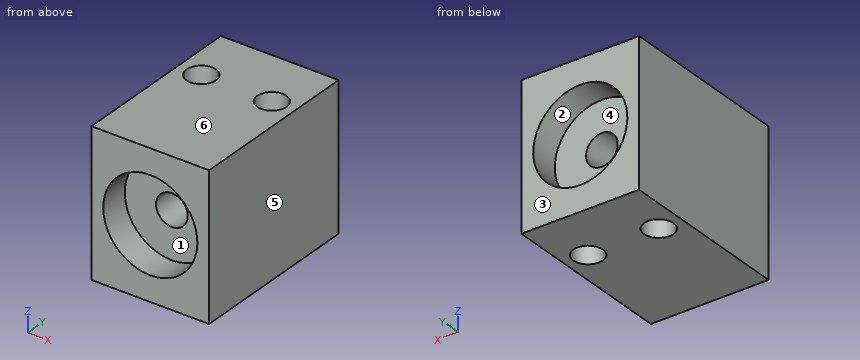
```python
from build123d import *

# Parameters (mm, degrees)
SKETCH1_W           = 20
SKETCH1_H           = 30
BOSS_EXTRUDE1_DEPTH = 12.25
SKETCH4_R           = 2.5
CUT_EXTRUDE1_DEPTH  = 25.5


with BuildPart() as part:
    # Sketch1 → Boss-Extrude1 (new body, symmetric)
    with BuildSketch(Plane.XY):
        Rectangle(SKETCH1_W, SKETCH1_H)
    extrude(amount=BOSS_EXTRUDE1_DEPTH, both=True)

    # Sketch3 → Cut-Revolve1 (revolve, cut)
    with BuildSketch(Plane(origin=(0, 0, 0), x_dir=(0, 0, -1), z_dir=(1, 0, 0))):
        Polygon((0, 15), (0, -15), (8, -15), (8, -10), (2.7, -10), (2.7, 10), (8, 10), (8, 15), align=None)
    revolve(axis=Axis((0, 15, 0), (0, -1, 0)), mode=Mode.SUBTRACT)

    # Sketch4 → Cut-Extrude1 (cut, through all)
    with BuildSketch(Plane(origin=(0, 0, -12.25), x_dir=(-1, 0, 0), z_dir=(0, 0, -1))):
        with Locations((-6, 5)):
            Circle(SKETCH4_R)
        with Locations((6, 5)):
            Circle(SKETCH4_R)
    extrude(amount=-CUT_EXTRUDE1_DEPTH, mode=Mode.SUBTRACT)


solid = part.part
```
Geometry: final body of the model. Coordinates: model frame, mm. Face numbers are marked on the shaded views. A direction names the side the tool comes from. Give positions to 0.01 mm unless a question says otherwise; leave off trailing zeros. Loops run counter-clockwise (first coordinate to the right, second up) from the corner with the lowest first, then second, coordinate; pieces in that order, holes last. Notation, with made-up numbers: (-17, 16.5) -> (42, 16.5) arc R26 cw to (42, 40.5) -> close; hole circle Ø1 at (59.5, -27). An arc over 180 degrees is marked (long way). Return JSON: item names as keys, results as strings.
Item 1: Section C-C, the plane y = -1.25. Output: boundary loops of the cut face in (x, z).
Filled in:
{"outline": "(-10, -12.25) -> (10, -12.25) -> (10, 12.25) -> (-10, 12.25) -> close; hole circle Ø5.4 at (0, 0)"}
Item 2: Line query: line 1 (X direction, y = 12.9, z = 0); line 2 (X direction, y = -5.5, z = 0); line 3 (X direction, y = 3, z = 10.75). Output: solid intervals per line, ascending.
Filled in:
{"line 1": "-10 to -8, 8 to 10", "line 2": "-10 to -2.7, 2.7 to 10", "line 3": "-10 to -7.5, -4.5 to 4.5, 7.5 to 10"}
Item 3: Mould query, pull axis Z, two halves, no side actions, for the marked faces 4, 5 and 6. Classes: released by +Z, released by -Z, zero draft, split by the parting line, or undercut.
Filled in:
{"face 4": "undercut", "face 5": "zero draft", "face 6": "released by +Z"}
Item 4: Section D-D, the plane z = -6.75. Output: boundary loops of the cut face in (x, y), plus the area to 3 significant figures.
Filled in:
{"outline": "(-10, -15) -> (-4.29, -15) -> (-4.29, -10) -> (4.29, -10) -> (4.29, -15) -> (10, -15) -> (10, 15) -> (4.29, 15) -> (4.29, 10) -> (-4.29, 10) -> (-4.29, 15) -> (-10, 15) -> close; hole circle Ø5 at (-6, 5); hole circle Ø5 at (6, 5)", "area": "475 mm^2"}
Item 5: Access query for the marked faces 1, 2 and 3. Directions: +Z, -Z, +X, -X, +Y, -Y. A direction counts if a zero-diameter tool reaches every point of the face in a straight line with its end or side. Return the directions, or none.
Filled in:
{"face 1": "-Y", "face 2": "+Y", "face 3": "+Z, -Z, +X, -X, +Y"}
Item 6: Section B-B, the plane x = 0. Output: boundary loops of the cut face in (y, z), plus the area to 3 significant figures.
Filled in:
{"outline": "(-15, -12.25) -> (15, -12.25) -> (15, -8) -> (10, -8) -> (10, -2.7) -> (-10, -2.7) -> (-10, -8) -> (-15, -8) -> close; (-15, 8) -> (-10, 8) -> (-10, 2.7) -> (10, 2.7) -> (10, 8) -> (15, 8) -> (15, 12.25) -> (-15, 12.25) -> close", "area": "467 mm^2"}
Item 7: Pin query (flat end, axial travel): P1, Ø4, axis at x = 6, y = 5, coming from the -Z side; P2, Ø5, axis at x = -0.5, z = 3.5, coming from the +Y side; P3, Ø5, axis at x = -1.5, z = -2.5, coming from the -Y side; P4, Ø2, axis at x = 6, z = -4, coming from the -Y side. Return the tip coordinate at first contact, or that it passes through.
Filled in:
{"P1": "through", "P2": "y = 10", "P3": "y = -10", "P4": "y = -15"}
Item 8: Section A-A, the plane z = 0. Output: boundary loops of the cut face in (x, y), plus the area to 3 significant figures.
Filled in:
{"outline": "(-10, -15) -> (-8, -15) -> (-8, -10) -> (-2.7, -10) -> (-2.7, 10) -> (-8, 10) -> (-8, 15) -> (-10, 15) -> close; (2.7, -10) -> (8, -10) -> (8, -15) -> (10, -15) -> (10, 15) -> (8, 15) -> (8, 10) -> (2.7, 10) -> close; hole circle Ø5 at (-6, 5); hole circle Ø5 at (6, 5)", "area": "293 mm^2"}
